Build history of the part. All positions in model axes, mm. Round coordinates to 2 decimals unless told otherwise and drop trailing zeros. Write each loop counter-clockwise with the first axis right and the second up, starting at its lowest first coordinate (ties: lowest second). Pieces come first, ordered by that corner, then holes.
1) Wall check: probe 1 along X at (y, z) = (38, 4.5); probe 2 along X at (y, z) = (73.5, 9.25); probe 3 along Y at (x, z) = (-106, 2.5). Give the ranges that are in metal, low to high.
2) Saw through at C-C (x = -257). Write the cut outline in (y, z).
3) Flat gauge pins, fed straight in: pin 1 (6.5 mm diameter, centred on x = -19.7, y = 50.57, fed in from -Z); pin 2 (3 mm diameter, centred on y = 29, z = 8, fed in from +X); pin 3 (2 mm diameter, centred on y = 41.5, z = 8.5, fed in from -X). Where does each tip first touch, or does it go through?
4) Saw through at A-A (x = -178.03). Write the cut outline in (y, z), plus the area to 3 significant figures.
5) Saw through at B-B (z = 8.25). Write the cut outline in (x, y), plus the area to 3 significant figures.
6) Pull direction X, two halves, no side cores. Call faces 1 (the cylindrical face through (-20.898, 46.755, 4.93)), 2 (the cylindrical face through (-423.663, 51.091, 4.93)), 3 (the flat face through (-217, 100.57, 5)), 4 (the cylindrical face through (30.29, 51.67, 4.93)): +X half, -X half, draft (parallel to the pull), parting line (faces both ways), or undercut.
7) Saw through at D-D (y = 83). Write the cut outline in (x, z).
Autodesk Inventor part; units mm, degrees
ref_plane "YZ Plane" through (0, 0, 0) normal (1, 0, 0) x (0, 1, 0)
ref_plane "XZ Plane" through (0, 0, 0) normal (0, 1, 0) x (-1, 0, 0)
ref_plane "XY Plane" through (0, 0, 0) normal (0, 0, 1) x (1, 0, 0)
sketch "Sketch1" plane through (0, 0, 0) normal (0, 0, 1) x (1, 0, 0)
  line L0 (-419.6966, 0.5698) -> (-19.6966, 0.5698)
  line L1 (-19.6966, 0.5698) -> (-19.6966, 100.5698)
  line L2 (-19.6966, 100.5698) -> (-419.6966, 100.5698)
  line L3 (-419.6966, 100.5698) -> (-419.6966, 0.5698)
  circle A0 centre (-419.6966, 50.5698) radius 50
  circle A1 centre (-19.6966, 50.5698) radius 50
  dimension "d12" = 400
  dimension "d13" = 100
  dimension "d14" = 100
  dimension "d15" = 100
extrude "Extrusion1" add sketch "Sketch1" along normal blind 10
sketch "Sketch2" plane through (0, 0, 10) normal (0, 0, 1) x (1, 0, 0)
  arc A0 (-419.6966, 100.5698) -> (-419.6966, 0.5698) centre (-419.6966, 50.5698) ccw
  arc A1 (-19.6966, 0.5698) -> (-19.6966, 100.5698) centre (-19.6966, 50.5698) ccw
  point P0 (0, 0)
hole "Hole1" at (-419.6966, 50.5698, 10) at (-19.6966, 50.5698, 10) direction (0, 0, -1) diameter 8 end through all
sketch "Sketch3" plane through (0, 0, 10) normal (0, 0, 1) x (1, 0, 0)
  circle A0 centre (-19.6966, 50.5698) radius 4
  circle A1 centre (-419.6966, 50.5698) radius 4
  line L0 (-19.6966, 0.5698) -> (-419.6966, 0.5698)
  circle A2 centre (-344.6966, 50.5698) radius 25
  circle A3 centre (-261.3633, 50.5698) radius 25
  circle A4 centre (-178.03, 50.5698) radius 25
  circle A5 centre (-94.6966, 52.8735) radius 25
  point P0 (0, 0)
  dimension "d16" = 50
  dimension "d17" = 50
  dimension "d18" = 50
  dimension "d19" = 50
  dimension "d20" = 83.3333
  dimension "d21" = 83.3333
  dimension "d22" = 83.3333
  dimension "d23" = 50
  dimension "d24" = 75
  dimension "d25" = 400
extrude "Extrusion2" cut sketch "Sketch3" against normal through all contours A2 | A3 | A4 | A5
equation "\"d14\" = d13"
equation "\"d15\" = d13"
equation "\"d17\" = d16"
equation "\"d18\" = d16"
equation "\"d19\" = d16"
equation "\"d20\" = -0.666667 * d24 + 0.333333 * d25"
equation "\"d21\" = d20"
equation "\"d22\" = d20"
properties part number "outer drive side"
Evaluation:
1. probe 1: x = -468.09 to -366.31, -323.09 to -282.97, -239.75 to -199.64, -156.42 to -114.79, -74.6 to 28.7
1. probe 2: x = -464.13 to -354.66, -334.74 to -271.32, -251.4 to -187.99, -168.07 to -108.82, -80.57 to 24.74
1. probe 3: y = 0.57 to 30.57, 75.17 to 100.57
2. outline: (0.57, 0) - (25.95, 0) - (25.95, 10) - (0.57, 10) - close; (75.19, 0) - (100.57, 0) - (100.57, 10) - (75.19, 10) - close
3. pin 1: passes through
3. pin 2: stops at x = 26.1
3. pin 3: stops at x = -469.04
4. outline: (0.57, 0) - (25.57, 0) - (25.57, 10) - (0.57, 10) - close; (75.57, 0) - (100.57, 0) - (100.57, 10) - (75.57, 10) - close
4. area: 500 mm2
5. outline: (-419.7, 0.57) - (-19.7, 0.57) arc R50 ccw to (-19.7, 100.57) - (-419.7, 100.57) arc R50 ccw to start; hole circle Ø8 at (-419.7, 50.57); hole circle Ø50 at (-344.7, 50.57); hole circle Ø50 at (-261.36, 50.57); hole circle Ø50 at (-178.03, 50.57); hole circle Ø50 at (-94.7, 52.87); hole circle Ø8 at (-19.7, 50.57)
5. area: 39,900 mm2
6. face 1: undercut
6. face 2: undercut
6. face 3: draft
6. face 4: +X half
7. outline: (-457.75, 0) - (18.36, 0) - (18.36, 10) - (-457.75, 10) - close
